For this review, take the finished solid that the model builds, in its own axes (mm). Face numbers are marked on the shaded views. A direction names the side the tool comes from. Coordinates: 2 decimals unless noted, no trailing zeros. Loops run counter-clockwise (first coordinate to the right, second up) from the corner with the lowest first, then second, coordinate; pieces in that order, holes last. Notation, with made-up numbers: (6.25, 70) -> (42.25, 70) arc R18 ccw to (42.25, 86) -> close; hole circle Ø11 at (85.25, 15). An arc over 180 degrees is marked (long way). Answer in a Markdown table with one row per item.
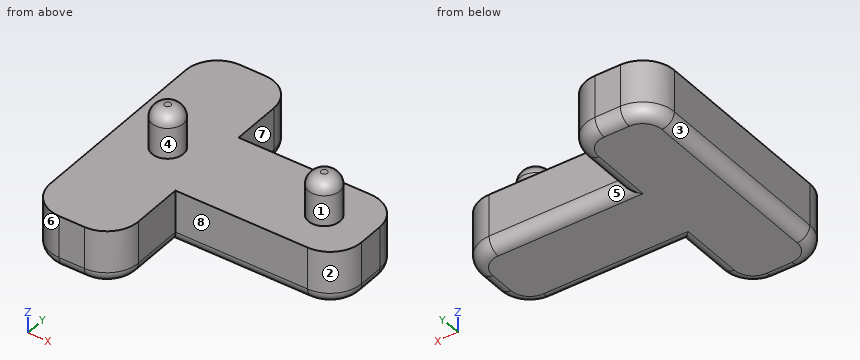
from build123d import *

# Parameters (mm, degrees)
F0_W     = 17.78
F0_H     = 17.78
F1_DEPTH = 11.049
F2_R     = 2.54
F3_R     = 3.175
F4_DEPTH = 8.763
F5_R     = 2.54


with BuildPart() as f1:
    # F0 (on Top) → F1 (new body)
    with BuildSketch(Plane.XY):
        with Locations((-16.51, 0)):
            Rectangle(F0_W, F0_H)
        with BuildLine():
            Line((-7.62, -19.303608), (-7.62, -8.89))
            Line((-7.62, -8.89), (-25.4, -8.89))
            Line((-25.4, -8.89), (-25.4, -19.303608))
            ThreePointArc((-25.4, -19.303608), (-23.540128, -23.793736), (-19.05, -25.653608))
            Line((-19.05, -25.653608), (-13.97, -25.653608))
            ThreePointArc((-13.97, -25.653608), (-9.479872, -23.793736), (-7.62, -19.303608))
        make_face()
        with BuildLine():
            Line((-25.4, 8.89), (-7.62, 8.89))
            Line((-7.62, 8.89), (-7.62, 18.796392))
            ThreePointArc((-7.62, 18.796392), (-9.479872, 23.28652), (-13.97, 25.146392))
            Line((-13.97, 25.146392), (-19.05, 25.146392))
            ThreePointArc((-19.05, 25.146392), (-23.540128, 23.28652), (-25.4, 18.796392))
            Line((-25.4, 18.796392), (-25.4, 8.89))
        make_face()
        with BuildLine():
            Line((-7.62, -8.89), (19.05, -8.89))
            ThreePointArc((19.05, -8.89), (23.540128, -7.030128), (25.4, -2.54))
            Line((25.4, -2.54), (25.4, 2.54))
            ThreePointArc((25.4, 2.54), (23.540128, 7.030128), (19.05, 8.89))
            Line((19.05, 8.89), (-7.62, 8.89))
            Line((-7.62, 8.89), (-7.62, -8.89))
        make_face()
    extrude(amount=F1_DEPTH)

    # F2
    f2_edges = [f1.edges().sort_by_distance(p)[0] for p in [
        (-7.62, -14.096804, 0),
        (5.715, -8.89, 0),
        (23.540128, -7.030128, 0),
    ]]
    fillet(f2_edges, radius=F2_R)

    # F3 (on face) → F4 (join)
    with BuildSketch(Plane.XY.offset(11.049)):
        with Locations((16.021419, 0)):
            Circle(F3_R)
        with Locations((-15.5448, 0)):
            Circle(F3_R)
    extrude(amount=F4_DEPTH)

    # F5
    f5_edges = [f1.edges().sort_by_distance(p)[0] for p in [
        (-18.7198, 0, 19.812),
        (12.846419, 0, 19.812),
    ]]
    fillet(f5_edges, radius=F5_R)


solid = f1.part
Item 1: Take a section at B-B, the plane z = 11.75. State the section outline as (x, y) points (3 decimals).
Worked answers:
| item | result |
|---|---|
| outline | circle Ø6.35 at (-15.545, 0); circle Ø6.35 at (16.021, 0) |
Item 2: The part is to be moulded in two halves that separate along X. For the marked faces 1, 2 and 3, say which applies: +X half, -X half, draft (parallel to the pull), parting line (faces both ways), or undercut.
Worked answers:
| item | result |
|---|---|
| face 1 | undercut |
| face 2 | +X half |
| face 3 | -X half |
Item 3: For L1, parallel to Y at x = 8, z = 10.5; L2, parallel to Z at x = -15, y = 20.5; L3, parallel to X at y = -0.5, z = 17.75, list the stretches that pass through material, from the lowest coordinate up.
Worked answers:
| item | result |
|---|---|
| L1 | -8.89 to 8.89 |
| L2 | 0 to 11.05 |
| L3 | -18.63 to -12.46, 12.93 to 19.11 |
Item 4: Take a section at A-A, the plane y = -14. State the section outline as (x, z) points, and give its area (3 significant figures).
Worked answers:
| item | result |
|---|---|
| outline | (-25.4, 2.54) arc R2.54 ccw to (-22.86, 0) -> (-10.16, 0) arc R2.54 ccw to (-7.62, 2.54) -> (-7.62, 11.05) -> (-25.4, 11.05) -> close |
| area | 194 mm² |
Item 5: For the marked faces 4, 5, 6, 7 and 8, list the 3-axis set-ups (+Z, -Z, +X, -X, +Y, -Y) from which the entire face can be reached by the end or side of a thin tool; tool diameter is ignored.
Worked answers:
| item | result |
|---|---|
| face 4 | +Z |
| face 5 | -Z, +X, +Y |
| face 6 | +Z, -Z, -X, -Y |
| face 7 | +Z, -Z, +X, +Y |
| face 8 | +Z, -Z, +X, -Y |
Item 6: Insertion check: pin 1 (10 mm diameter, centred on x = -13.5, z = 5.5, fed in from -Y); pin 2 (3 mm diameter, centred on y = 19, z = 3.5, fed in from +X); pin 3 (1.5 mm diameter, centred on y = -2.5, z = 14.5, fed in from -X); pin 4 (4 mm diameter, centred on x = 18.5, z = 17, fed in from +Y). Each pin has a flat end and moves straight along its axis. Give the tip position at first contact, or say it passes through.
Worked answers:
| item | result |
|---|---|
| pin 1 | y = -25.65 |
| pin 2 | x = -7.62 |
| pin 3 | x = -18.19 |
| pin 4 | y = 3.14 |
Item 7: Take a section at C-C, the plane x = -5. State the section outline as (y, z) points, and give its area (3 significant figures).
Worked answers:
| item | result |
|---|---|
| outline | (-8.89, 2.54) arc R2.54 ccw to (-6.35, 0) -> (6.35, 0) arc R2.54 ccw to (8.89, 2.54) -> (8.89, 11.05) -> (-8.89, 11.05) -> close |
| area | 194 mm² |
